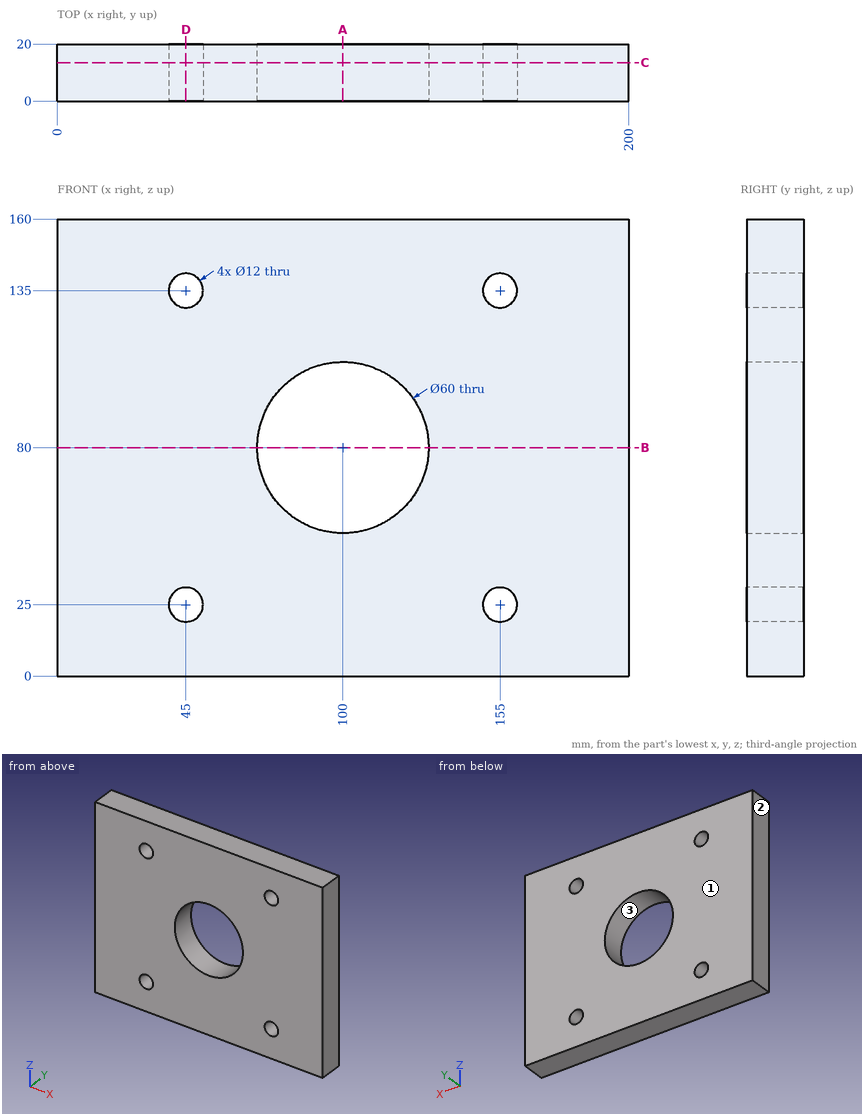
For this review, use the dimensioned drawing (mm, ordinates from the lowest corner) and the shaded views. Round coordinates to 2 decimals unless told otherwise and drop trailing zeros. Write each loop counter-clockwise with the first axis right and the second up, starting at its lowest first coordinate (ties: lowest second). Pieces come first, ordered by that corner, then holes. Notation, with made-up numbers: (69.5, 20) -> (106.5, 20) arc R35 cw to (106.5, 54) -> close; hole circle Ø1 at (-1, 32). An arc over 180 degrees is marked (long way). Use one line per item in the form item = value.
Q1. Consider section D-D (x = 45). State the section outline as (y, z) points, then the cut area to 3 significant figures.
Resolved:
outline = (0, 0) -> (20, 0) -> (20, 19) -> (0, 19) -> close; (0, 31) -> (20, 31) -> (20, 129) -> (0, 129) -> close; (0, 141) -> (20, 141) -> (20, 160) -> (0, 160) -> close
area = 2,720 mm²
Q2. Consider section B-B (z = 80). State the section outline as (x, y) points.
Resolved:
outline = (0, 0) -> (70, 0) -> (70, 20) -> (0, 20) -> close; (130, 0) -> (200, 0) -> (200, 20) -> (130, 20) -> close
Q3. The part is to be moulded in two halves that separate along X. For the marked faces 1, 2 and 3, say which applies: released by +X, released by -X, zero draft, split by the parting line, or undercut.
Resolved:
face_1 = zero draft
face_2 = released by -X
face_3 = undercut
Q4. Consider section C-C (y = 13.5). State the section outline as (x, z) points, then the cut area to 3 significant figures.
Resolved:
outline = (0, 0) -> (200, 0) -> (200, 160) -> (0, 160) -> close; hole circle Ø12 at (45, 25); hole circle Ø12 at (45, 135); hole circle Ø60 at (100, 80); hole circle Ø12 at (155, 25); hole circle Ø12 at (155, 135)
area = 28,700 mm²
Q5. To check wall thickness, follow probe 1 along X at (y, z) = (14.75, 135); probe 2 along Z at (x, y) = (100, 8.25); probe 3 along X at (y, z) = (16, 30.5). State the ranges of each line that lie inside material, in increasing order. Write a range as from..to.
Resolved:
probe_1 = 0..39, 51..149, 161..200
probe_2 = 0..50, 110..160
probe_3 = 0..42.6, 47.4..152.6, 157.4..200
Q6. Consider section A-A (x = 100). State the section outline as (y, z) points.
Resolved:
outline = (0, 0) -> (20, 0) -> (20, 50) -> (0, 50) -> close; (0, 110) -> (20, 110) -> (20, 160) -> (0, 160) -> close
